Check sheet for the modelled part. Datum: model origin and axes. Units: mm. Face numbers are marked on the shaded views. A direction names the side the tool comes from. Round coordinates to 2 decimals unless told otherwise and drop trailing zeros. Write each loop counter-clockwise with the first axis right and the second up, starting at its lowest first coordinate (ties: lowest second). Pieces come first, ordered by that corner, then holes. Notation, with made-up numbers: M 21.25,27 L 51.25,27 A13 cw 51.25,37 Z; hole C 25,47.5 d6. An arc over 180 degrees is marked long. Answer in a Markdown table with one row per item.
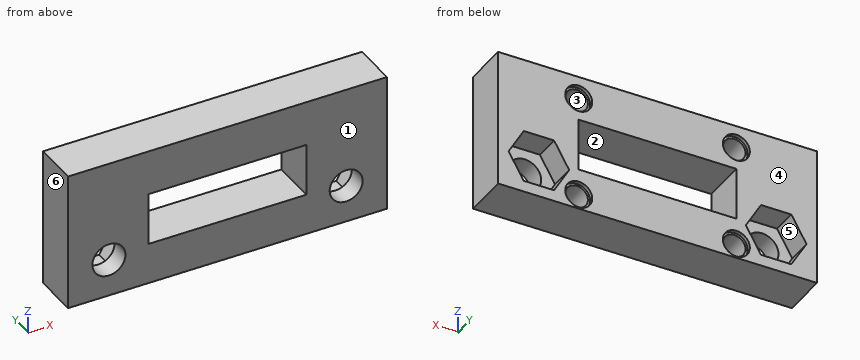
```python
from build123d import *

# Parameters (mm, degrees)
BOSS_EXTRUDE1_DEPTH = 8
SKETCH2_R           = 2.2
CUT_EXTRUDE1_DEPTH  = 20
CUT_EXTRUDE2_DEPTH  = 5.3
SKETCH4_R           = 1.5
CUT_EXTRUDE3_DEPTH  = 4
SKETCH5_R           = 1.8
CUT_EXTRUDE4_DEPTH  = 0.5
CUT_EXTRUDE5_DEPTH  = 3.4
CUT_EXTRUDE6_DEPTH  = 18.4
SKETCH9_W           = 21
SKETCH9_H           = 3
CUT_EXTRUDE8_DEPTH  = 2


with BuildPart() as part:
    # Sketch1 → Boss-Extrude1 (new body)
    with BuildSketch(Plane(origin=(0, 0, 0), x_dir=(1, 0, 0), z_dir=(0, 1, 0))):
        Polygon((-21.25, -18.5), (21.25, -18.5), (21.25, 0), (15.81, 0), (-15.81, 0), (-21.25, 0), align=None)
    extrude(amount=BOSS_EXTRUDE1_DEPTH)

    # Sketch2 → Cut-Extrude1 (cut)
    with BuildSketch(Plane(origin=(0, 8, 0), x_dir=(1, 0, 0), z_dir=(0, 1, 0))):
        with Locations((-15.81, -5)):
            Circle(SKETCH2_R)
        with Locations((15.81, -5)):
            Circle(SKETCH2_R)
    extrude(amount=-CUT_EXTRUDE1_DEPTH, mode=Mode.SUBTRACT)

    # Sketch3 → Cut-Extrude2 (cut)
    with BuildSketch(Plane(origin=(0, 8, 0), x_dir=(1, 0, 0), z_dir=(0, 1, 0))):
        with BuildLine():
            ThreePointArc((-10.5, -14.4), (-11.277817459, -16.277817459), (-9.4, -15.5))
            Line((-9.4, -15.5), (-10.5, -15.5))
            Line((-10.5, -15.5), (-10.5, -14.4))
        make_face()
        with BuildLine():
            Line((-10.5, -15.5), (-9.4, -15.5))
            ThreePointArc((-9.4, -15.5), (-9.722182541, -14.722182541), (-10.5, -14.4))
            Line((-10.5, -14.4), (-10.5, -15.5))
        make_face()
        with BuildLine():
            ThreePointArc((-9.4, -2), (-11.277817459, -1.222182541), (-10.5, -3.1))
            Line((-10.5, -3.1), (-10.5, -2))
            Line((-10.5, -2), (-9.4, -2))
        make_face()
        with BuildLine():
            Line((-10.5, -2), (-10.5, -3.1))
            ThreePointArc((-10.5, -3.1), (-9.722182541, -2.777817459), (-9.4, -2))
            Line((-9.4, -2), (-10.5, -2))
        make_face()
        with BuildLine():
            ThreePointArc((9.4, -2), (9.722182541, -2.777817459), (10.5, -3.1))
            Line((10.5, -3.1), (10.5, -2))
            Line((10.5, -2), (9.4, -2))
        make_face()
        with BuildLine():
            Line((10.5, -2), (10.5, -3.1))
            ThreePointArc((10.5, -3.1), (11.277817459, -2.777817459), (11.6, -2))
            ThreePointArc((11.6, -2), (10.5, -0.9), (9.4, -2))
            Line((9.4, -2), (10.5, -2))
        make_face()
        with BuildLine():
            Line((10.5, -16.6), (10.5, -15.5))
            Line((10.5, -15.5), (9.4, -15.5))
            ThreePointArc((9.4, -15.5), (9.722182541, -16.277817459), (10.5, -16.6))
        make_face()
        with BuildLine():
            Line((10.5, -14.4), (10.5, -15.5))
            Line((10.5, -15.5), (10.5, -16.6))
            ThreePointArc((10.5, -16.6), (11.277817459, -16.277817459), (11.6, -15.5))
            ThreePointArc((11.6, -15.5), (11.277817459, -14.722182541), (10.5, -14.4))
        make_face()
        with BuildLine():
            Line((9.4, -15.5), (10.5, -15.5))
            Line((10.5, -15.5), (10.5, -14.4))
            ThreePointArc((10.5, -14.4), (9.722182541, -14.722182541), (9.4, -15.5))
        make_face()
    extrude(amount=-CUT_EXTRUDE2_DEPTH, mode=Mode.SUBTRACT)

    # Sketch4 → Cut-Extrude3 (cut)
    with BuildSketch(Plane(origin=(0, 8, 0), x_dir=(1, 0, 0), z_dir=(0, 1, 0))):
        with Locations((-10.5, -2)):
            Circle(SKETCH4_R)
        with Locations((10.5, -2)):
            Circle(SKETCH4_R)
        with Locations((-10.5, -15.5)):
            Circle(SKETCH4_R)
        with Locations((10.5, -15.5)):
            Circle(SKETCH4_R)
    extrude(amount=-CUT_EXTRUDE3_DEPTH, mode=Mode.SUBTRACT)

    # Sketch5 → Cut-Extrude4 (cut)
    with BuildSketch(Plane(origin=(0, 8, 0), x_dir=(1, 0, 0), z_dir=(0, 1, 0))):
        with Locations((-10.5, -2)):
            Circle(SKETCH5_R)
        with Locations((10.5, -2)):
            Circle(SKETCH5_R)
        with Locations((-10.5, -15.5)):
            Circle(SKETCH5_R)
        with Locations((10.5, -15.5)):
            Circle(SKETCH5_R)
    extrude(amount=-CUT_EXTRUDE4_DEPTH, mode=Mode.SUBTRACT)

    # Sketch6 → Cut-Extrude5 (cut)
    with BuildSketch(Plane(origin=(0, 8, 0), x_dir=(1, 0, 0), z_dir=(0, 1, 0))):
        Polygon((-11.768548116, -5), (-13.789274058, -1.5), (-17.830725942, -1.5), (-19.851451884, -5), (-17.830725942, -8.5), (-13.789274058, -8.5), align=None)
        Polygon((19.851451884, -5), (17.830725942, -1.5), (13.789274058, -1.5), (11.768548116, -5), (13.789274058, -8.5), (17.830725942, -8.5), align=None)
    extrude(amount=-CUT_EXTRUDE5_DEPTH, mode=Mode.SUBTRACT)

    # Sketch7 → Cut-Extrude6 (cut)
    with BuildSketch(Plane(origin=(0, 8, 0), x_dir=(1, 0, 0), z_dir=(0, 1, 0))):
        Polygon((10.5, -9), (10.5, -5.5), (-10.5, -5.5), (-10.5, -12.5), (10.5, -12.5), align=None)
    extrude(amount=-CUT_EXTRUDE6_DEPTH, mode=Mode.SUBTRACT)

    # Sketch9 → Cut-Extrude8 (cut)
    with BuildSketch(Plane.XZ):
        Polygon((-10.5, 15.5), (10.5, 15.5), (10.5, 18.5), (-21.25, 18.5), (-21.25, 0), (-15.81, 0), (0, 0), (0, 2), (-10.5, 2), (-10.5, 5.5), (-10.5, 12.5), align=None)
        with BuildLine():
            ThreePointArc((-13.61, 5), (-14.254365081, 3.444365081), (-15.81, 2.8))
            ThreePointArc((-15.81, 2.8), (-17.365634919, 6.555634919), (-13.61, 5))
        make_face(mode=Mode.SUBTRACT)
        with Locations((0, 14)):
            Rectangle(SKETCH9_W, SKETCH9_H)
        Polygon((10.5, 2), (10.5, 5.5), (-10.5, 5.5), (-10.5, 2), (0, 2), align=None)
        Polygon((10.5, 18.5), (10.5, 15.5), (10.5, 12.5), (10.5, 5.5), (10.5, 2), (0, 2), (0, 0), (15.81, 0), (21.25, 0), (21.25, 18.5), align=None)
        with BuildLine():
            ThreePointArc((18.01, 5), (17.365634919, 3.444365081), (15.81, 2.8))
            ThreePointArc((15.81, 2.8), (14.254365081, 6.555634919), (18.01, 5))
        make_face(mode=Mode.SUBTRACT)
    extrude(amount=-CUT_EXTRUDE8_DEPTH, mode=Mode.SUBTRACT)


solid = part.part
```
1. Section check A-A, the plane x = -6. Record the cut outline in (y, z).
Found:
| item | result |
|---|---|
| outline | M 2,0 L 8,0 L 8,5.5 L 2,5.5 Z; M 2,12.5 L 8,12.5 L 8,18.5 L 2,18.5 Z |
2. Section check B-B, the plane y = 6.55. Record the cut outline in (x, z).
Found:
| item | result |
|---|---|
| outline | M -21.25,0 L 21.25,0 L 21.25,18.5 L -21.25,18.5 Z; hole M -19.85,5 L -17.83,1.5 L -13.79,1.5 L -11.77,5 L -13.79,8.5 L -17.83,8.5 Z; hole C -10.5,2 d3; hole C -10.5,15.5 d3; hole M -10.5,5.5 L 10.5,5.5 L 10.5,12.5 L -10.5,12.5 Z; hole C 10.5,2 d3; hole C 10.5,15.5 d3; hole M 11.77,5 L 13.79,1.5 L 17.83,1.5 L 19.85,5 L 17.83,8.5 L 13.79,8.5 Z |
3. Access from +Z, -Z, +X, -X, +Y, -Y to the whole of each face (thin tool, end or side, straight path). Record for the marked faces 1, 2 and 3.
Found:
| item | result |
|---|---|
| face 1 | +Z, -Z, +X, -X, -Y |
| face 2 | +Y, -Y |
| face 3 | +Y |
4. Scan lines: L1, parallel to X at y = 7.8, z = 15.5; L2, parallel to X at y = 3.3, z = 15.5; L3, parallel to Z at x = 15.81, y = 4. Record each from-to range of solid material in increasing order.
Found:
| item | result |
|---|---|
| L1 | x = -21.25 to -12.3, -8.7 to 8.7, 12.3 to 21.25 |
| L2 | x = -21.25 to -11.6, -9.4 to 9.4, 11.6 to 21.25 |
| L3 | z = 0 to 2.8, 7.2 to 18.5 |
5. Draft check along X on the marked faces 4, 5 and 6. Enter one of: +X half, -X half, draft (parallel to the pull), parting line (faces both ways), or undercut.
Found:
| item | result |
|---|---|
| face 4 | draft |
| face 5 | undercut |
| face 6 | -X half |
6. Go/stop test with flat-tipped pins: pin 1 (0.9 mm diameter, centred on x = -10.5, z = 2, fed in from +Y); pin 2 (2.5 mm diameter, centred on x = -10.5, z = 2, fed in from +Y); pin 3 (2 mm diameter, centred on x = -2, z = 7.5, fed in from -Y); pin 4 (2.5 mm diameter, centred on x = -10.5, z = 15, fed in from +Y). Record where each tip stops, or that it passes through.
Found:
| item | result |
|---|---|
| pin 1 | stops at y = 2.7 |
| pin 2 | stops at y = 4 |
| pin 3 | passes through |
| pin 4 | stops at y = 7.5 |
7. Section check D-D, the plane x = -15.81. Record the cut outline in (y, z).
Found:
| item | result |
|---|---|
| outline | M 2,0 L 8,0 L 8,1.5 L 4.6,1.5 L 4.6,2.8 L 2,2.8 Z; M 2,7.2 L 4.6,7.2 L 4.6,8.5 L 8,8.5 L 8,18.5 L 2,18.5 Z |
8. Section check C-C, the plane z = 6.5. Record the cut outline in (x, y), and give its area (3 significant figures).
Found:
| item | result |
|---|---|
| outline | M -21.25,2 L -17.42,2 L -17.42,4.6 L -18.99,4.6 L -18.99,8 L -21.25,8 Z; M -14.2,2 L -10.5,2 L -10.5,8 L -12.63,8 L -12.63,4.6 L -14.2,4.6 Z; M 10.5,2 L 14.2,2 L 14.2,4.6 L 12.63,4.6 L 12.63,8 L 10.5,8 Z; M 17.42,2 L 21.25,2 L 21.25,8 L 18.99,8 L 18.99,4.6 L 17.42,4.6 Z |
| area | 69.1 mm2 |
